Input: part model. Units: mm. Frame: model coordinates. Face numbers are marked on the shaded views. A direction names the side the tool comes from. Round coordinates to 2 decimals unless told otherwise and drop trailing zeros. Loops run counter-clockwise (first coordinate to the right, second up) from the corner with the lowest first, then second, coordinate; pieces in that order, holes last.
(1) Access query for the marked faces 1, 2 and 3. Directions: +Z, -Z, +X, -X, +Y, -Y. A direction counts if a zero-diameter tool reaches every point of the face in a straight line with its end or side. Return the directions, or none.
(2) Cut plane A-A, the plane x = -35.5. Output: boundary loops of the cut face in (y, z).
(3) Line query: line 1 (Y direction, x = -13, z = -46); line 2 (Z direction, x = -15, y = 99); line 3 (Y direction, x = -20.5, z = 38.5). Output: solid intervals per line, ascending.
(4) Cut plane D-D, the plane y = 47. Output: boundary loops of the cut face in (x, z), and give its area (3 significant figures).
(5) Cut plane B-B, the plane y = -38.5. Output: boundary loops of the cut face in (x, z), and give its area (3 significant figures).
(6) First-contact query: pin 1 Ø2 at (y, z) = (26, 55.5) entering from -X; pin 2 Ø3 at (y, z) = (-20.5, 37.5) entering from +X; pin 3 Ø5 at (x, z) = (-33.5, -16) entering from -Y. Flat tips, straight axial feed; report the tip coordinate or a pass-through.
(7) Cut plane C-C, the plane z = -12. Output: boundary loops of the cut face in (x, y), and give its area (3 significant figures).
from build123d import *

# Parameters (mm, degrees)
F0_R          = 82
F1_DEPTH      = 25
F1_DEPTH_BACK = 149
F2_R          = 28.575
F3_DEPTH      = 174.001
F6_DEPTH      = 33
F7_R          = 44.45
F7_R_2        = 28.575
F8_DEPTH      = 78
F10_DEPTH     = 174.001


with BuildPart() as f1:
    # F0 (on Front) → F1 (new body, two sides)
    with BuildSketch(Plane.XZ) as f1_sk:
        Circle(F0_R)
    extrude(amount=F1_DEPTH)
    extrude(f1_sk.sketch, amount=-F1_DEPTH_BACK)

    # F2 (on face) → F3 (cut, through all)
    with BuildSketch(Plane.XZ.offset(25)):
        Circle(F2_R)
    extrude(amount=-F3_DEPTH, mode=Mode.SUBTRACT)

    # F4 (on face) → F6 (join)
    with BuildSketch(Plane.XZ.offset(25)):
        with BuildLine():
            ThreePointArc((-32.0991935027, 75.4562242395), (-64.6168817958, 50.4842409767), (-80.9803496399, 12.8911974698))
            Line((-80.9803496399, 12.8911974698), (-64.4803693095, 0))
            Line((-64.4803693095, 0), (-15.8976419198, 62.7981848607))
            Line((-15.8976419198, 62.7981848607), (-32.0991935027, 75.4562242395))
        make_face()
    extrude(amount=F6_DEPTH)

    # F7 (on face) → F8 (cut)
    with BuildSketch(Plane.XZ.offset(25)):
        Circle(F7_R)
        Circle(F7_R_2, mode=Mode.SUBTRACT)
    extrude(amount=-F8_DEPTH, mode=Mode.SUBTRACT)

    # F9 (on face) → F10 (cut, through all)
    with BuildSketch(Plane.XZ.offset(25)):
        with BuildLine():
            Line((91, 95.2523052692), (0, 95.2523052692))
            Line((0, 95.2523052692), (0, 82))
            ThreePointArc((0, 82), (57.9827560573, 57.9827560573), (82, 0))
            ThreePointArc((82, 0), (54.3323108288, -61.4166101311), (-10, -81.3879597975))
            Line((-10, -81.3879597975), (-10, -94.1154360771))
            Line((-10, -94.1154360771), (91, -94.1154360771))
            Line((91, -94.1154360771), (91, 95.2523052692))
        make_face()
        with BuildLine():
            ThreePointArc((82, 0), (57.9827560573, 57.9827560573), (0, 82))
            Line((0, 82), (0, 28.575))
            ThreePointArc((0, 28.575), (20.2055762724, 20.2055762724), (28.575, 0))
            ThreePointArc((28.575, 0), (16.2908045381, -23.4763777551), (-10, -26.7680896778))
            Line((-10, -26.7680896778), (-10, -81.3879597975))
            ThreePointArc((-10, -81.3879597975), (54.3323108288, -61.4166101311), (82, 0))
        make_face()
    extrude(amount=-F10_DEPTH, mode=Mode.SUBTRACT)


solid = f1.part
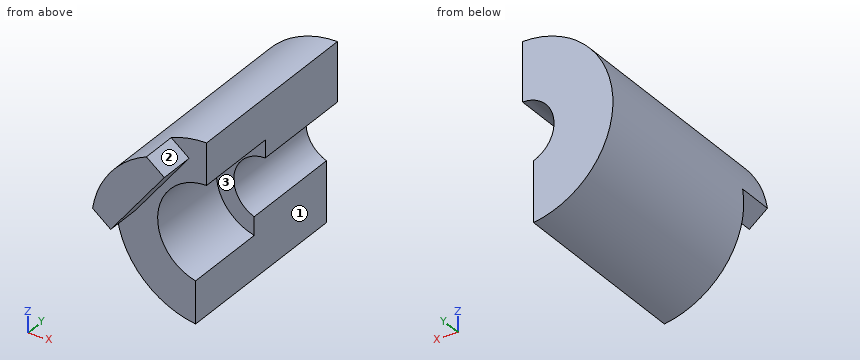
Reported:
1. face 1: -Z, +X, +Y, -Y
1. face 2: +Z, +X, -Y
1. face 3: +X, -Y
2. outline: (-58, 37.46) - (-25, 37.46) - (-25, 26.75) - (53, 26.75) - (53, -26.75) - (-25, -26.75) - (-25, -73.92) - (149, -73.92) - (149, 73.92) - (-58, 73.92) - close
3. line 1: y = -25 to 149
3. line 2: z = -80.62 to -24.32, 24.32 to 80.62
3. line 3: y = 53 to 149
4. outline: (-10, -81.39) - (-10, -43.31) arc R44.45 cw to (0, 44.45) - (0, 82) arc R82 ccw to start
4. area: 7,080 mm2
5. outline: (-80.98, 12.89) - (-64.48, 0) - (-15.9, 62.8) - (-32.1, 75.46) arc R82 ccw to start
5. area: 2,200 mm2
6. pin 1: stops at x = -61.27
6. pin 2: stops at x = -21.33
6. pin 3: stops at y = 53
7. outline: (-81.12, -25) - (-42.8, -25) - (-42.8, 53) - (-25.93, 53) - (-25.93, 149) - (-81.12, 149) - close
7. area: 8,290 mm2
